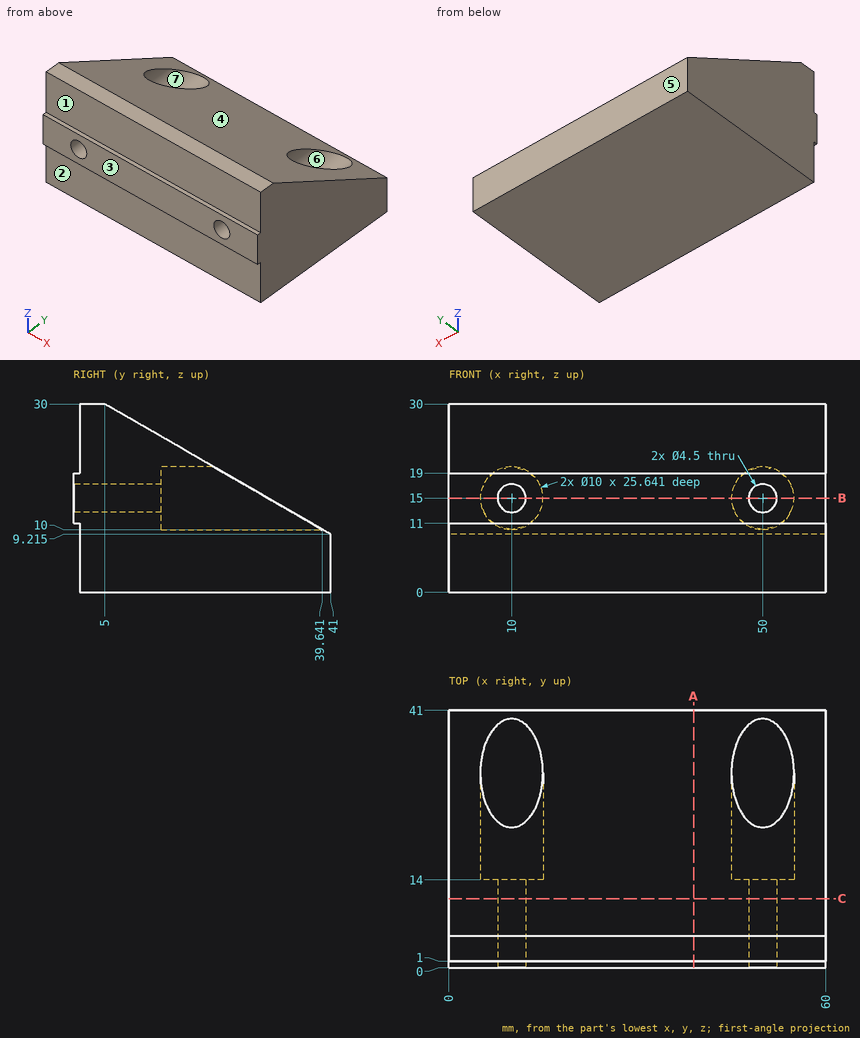
Can you work these out from the drawing? Everything is in mm from the part's minimum corner. A direction names the side the tool comes from. Round coordinates to 2 decimals unless told otherwise and drop trailing zeros. Loops run counter-clockwise (first coordinate to the right, second up) from the corner with the lowest first, then second, coordinate; pieces in that order, holes last. Notation, with made-up numbers: (-22.5, 74) -> (11.5, 74) arc R27 cw to (11.5, 108) -> close; hole circle Ø5 at (14.5, 61). An arc over 180 degrees is marked (long way). One line per question, with ' | ' between items.
(1) Thinking about a two-plate mould opening in Z: for the marked faces 4, 5, 6 and 7, which applies, released by +Z, released by -Z, zero draft, split by the parting line, or undercut?
Model answer:
face 4: released by +Z | face 5: zero draft | face 6: undercut | face 7: undercut
(2) If I drill on probe 1 along X at (y, z) = (8.25, 15); probe 2 along X at (y, z) = (25.5, 17.5); probe 3 along Y at (x, z) = (48, 4.5), over which ranges is the centre line in solid material (lowest first)?
Model answer:
probe 1: x = 0 to 7.75, 12.25 to 47.75, 52.25 to 60 | probe 2: x = 0 to 5.67, 14.33 to 45.67, 54.33 to 60 | probe 3: y = 1 to 41
(3) If we section it at A-A on x = 39: List the corners of the cut face in (y, z) for me (1 decimal), and give its area (3 significant figures).
Model answer:
outline: (0, 11) -> (1, 11) -> (1, 0) -> (41, 0) -> (41, 9.2) -> (5, 30) -> (1, 30) -> (1, 19) -> (0, 19) -> close | area: 834 mm^2
(4) For pin 1 Ø3.5 at (x, z) = (10, 15) entering from +Y; pin 2 Ø6 at (x, z) = (50, 15) entering from +Y; pin 3 Ø5 at (x, z) = (7.5, 13) entering from +Y (1 decimal); pin 4 Ø3 at (x, y) = (31, 8) entering from +Z (1 decimal), each with a flat end and sliding along its axis, tell me the tip position at first contact or that it passes through.
Model answer:
pin 1: passes through | pin 2: stops at y = 14 | pin 3: stops at y = 38.8 | pin 4: stops at z = 29.1
(5) For the marked faces 1, 2 and 3, which set-ups out of +Z, -Z, +X, -X, +Y, -Y let a thin tool reach every point of the face, with its end or its side?
Model answer:
face 1: +Z, +X, -X, -Y | face 2: -Z, +X, -X, -Y | face 3: +Z, -Z, +X, -X, -Y
(6) If we section it at C-C on y = 11: List the corners of the cut face in (x, z) for me.
Model answer:
outline: (0, 0) -> (60, 0) -> (60, 26.54) -> (0, 26.54) -> close; hole circle Ø4.5 at (10, 15); hole circle Ø4.5 at (50, 15)
(7) If we section it at B-B on z = 15: List the corners of the cut face in (x, y) for me, and give its area (3 significant figures).
Model answer:
outline: (0, 0) -> (7.75, 0) -> (7.75, 14) -> (5, 14) -> (5, 30.98) -> (0, 30.98) -> close; (12.25, 0) -> (47.75, 0) -> (47.75, 14) -> (45, 14) -> (45, 30.98) -> (15, 30.98) -> (15, 14) -> (12.25, 14) -> close; (52.25, 0) -> (60, 0) -> (60, 30.98) -> (55, 30.98) -> (55, 14) -> (52.25, 14) -> close | area: 1,390 mm^2
